Can you work these out from the model? Positions are in its coordinate system, mm. A direction names the side the tool comes from. Coordinates: 2 decimals unless noted, no trailing zeros. Order: outer loops, then holes, each group sorted by start corner. A loop starts at its lowest first (then second) coordinate and runs counter-clockwise, first axis right, second up. Notation, with made-up numbers: (25, -34) - (40, -34) arc R29 cw to (40, -2) - close; hole circle Ø3 at (-0.5, 9). An arc over 180 degrees is marked (long way). Use a Markdown table: item, result. Add a question column.
(1) We'd pull the mould along X, two halves only. Please class faces 3 (the flat face through (235.372, 15, 10)), 4 (the cylindrical face through (167.365, -129.391, 9.86)), 5 (the flat face through (-8, -175, 20)), 6 (the cylindrical face through (-176.777, 164.75, 9.86)): pulls with the +X half, pulls with the -X half, needs draft (parallel to the pull), parting line crosses it, or undercut.
(2) I want a section at A-A (y = -43). List the corners of the cut face in (x, z) for me, and give its area (3 significant figures).
(3) I want a section at B-B (z = 13.25). List the corners of the cut face in (x, y) for me.
(4) On a 3-axis mill with a long thin cutter (end or side, diameter ignored), from which of +Z, -Z, +X, -X, +Y, -Y can I reach the whole of each face in a straight line? I mean faces 1 (the cylindrical face through (-177, -129, 10)), 2 (the flat face through (-8, 237.757, 10)). Say none if no direction works.
(5) I want a section at C-C (x = 44.5). List the corners of the cut face in (y, z) for me.
(6) If I drill on L1, parallel to Y at x = 49, z = 8; L2, parallel to X at y = 63.5, z = 12; L3, parallel to X at y = 163, z = 18, over which ranges is the centre line in solid material (lowest first)? Write a range as [from, to].
```python
from build123d import *

# Parameters (mm, degrees)
F0_W     = 480
F0_H     = 440
F1_DEPTH = 20
F2_W     = 175
F2_H     = 150
F3_DEPTH = 20
F4_R     = 10


with BuildPart() as f1:
    # F0 (on Top) → F1 (new body)
    with BuildSketch(Plane.XY):
        with Locations((-4.628388, 17.757134)):
            Rectangle(F0_W, F0_H)
    extrude(amount=F1_DEPTH)

    # F2 (on face) → F3 (cut, through all)
    with BuildSketch(Plane.XY.offset(20)):
        with Locations((-92.128388, 92.757134)):
            Rectangle(F2_W, F2_H)
        with Locations((82.871612, 92.757134)):
            Rectangle(F2_W, F2_H)
        with Locations((-92.128388, -57.242866)):
            Rectangle(F2_W, F2_H)
        with Locations((82.871612, -57.242866)):
            Rectangle(F2_W, F2_H)
    extrude(amount=-F3_DEPTH, mode=Mode.SUBTRACT)

    # F4
    f4_edges = [f1.edges().sort_by_distance(p)[0] for p in [
        (-179.628388, 167.757134, 10),
        (-179.628388, -132.242866, 10),
        (170.371612, 167.757134, 10),
        (170.371612, -132.242866, 10),
    ]]
    fillet(f4_edges, radius=F4_R)


solid = f1.part
```
Answers follow:
| question | item | result |
|---|---|---|
| 1 | face 3 | pulls with the +X half |
| 1 | face 4 | undercut |
| 1 | face 5 | needs draft |
| 1 | face 6 | undercut |
| 2 | outline | (-244.63, 0) - (-179.63, 0) - (-179.63, 20) - (-244.63, 20) - close; (170.37, 0) - (235.37, 0) - (235.37, 20) - (170.37, 20) - close |
| 2 | area | 2,600 mm² |
| 3 | outline | (-244.63, -202.24) - (235.37, -202.24) - (235.37, 237.76) - (-244.63, 237.76) - close; hole (-179.63, -122.24) arc R10 ccw to (-169.63, -132.24) - (160.37, -132.24) arc R10 ccw to (170.37, -122.24) - (170.37, 157.76) arc R10 ccw to (160.37, 167.76) - (-169.63, 167.76) arc R10 ccw to (-179.63, 157.76) - close |
| 4 | face 1 | +Z, -Z |
| 4 | face 2 | +Z, -Z, +X, -X, +Y |
| 5 | outline | (-202.24, 0) - (-132.24, 0) - (-132.24, 20) - (-202.24, 20) - close; (167.76, 0) - (237.76, 0) - (237.76, 20) - (167.76, 20) - close |
| 6 | L1 | y = [-202.24, -132.24], [167.76, 237.76] |
| 6 | L2 | x = [-244.63, -179.63], [170.37, 235.37] |
| 6 | L3 | x = [-244.63, -178.14], [168.89, 235.37] |
